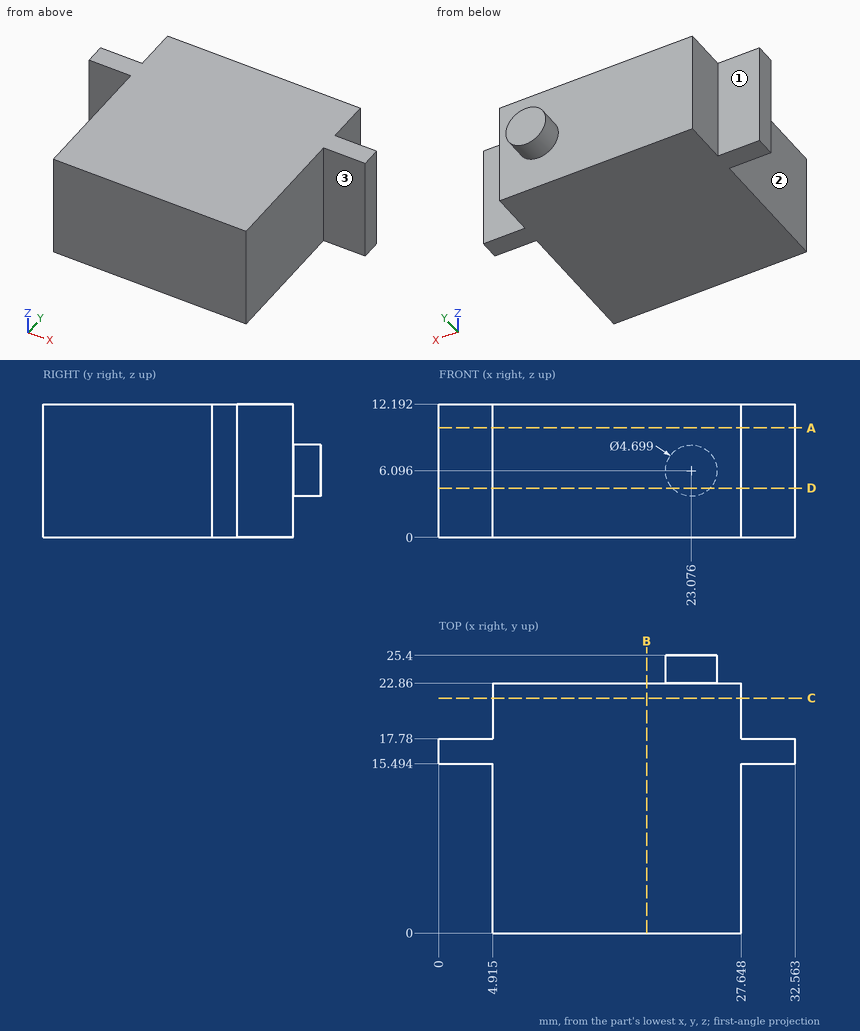
Print and shaded views of the part. All mm, measured from the part's lowest x, y and z. A direction names the side the tool comes from. Coordinates: 2 decimals unless noted, no trailing zeros. Write each loop counter-clockwise with the first axis right and the second up, starting at its lowest first coordinate (ties: lowest second). Pieces come first, ordered by that corner, then holes. Notation, with made-up numbers: M 7,22.25 L 24,22.25 A26 cw 24,56.25 Z; hole C 54.5,23 d5. An arc over 180 degrees is marked long. Return JSON: item names as keys, results as strings.
1. 3-axis set-ups, long thin cutter, end or side, ignore diameter. For the marked faces 1, 2 and 3: which of +Z, -Z, +X, -X, +Y, -Y reach the whole face in a straight line?
Determined:
{"face 1": "+Z, -Z, -X, +Y", "face 2": "+Z, -Z, -X, -Y", "face 3": "+Z, -Z, +X, -Y"}
2. Probe L1, parallel to X at y = 8.75, z = 1.5 (1 decimal); L2, parallel to Y at x = 17, z = 9.25; L3, parallel to Y at x = 29, z = 7.25. List the from-to ranges inside material, lowest first.
Determined:
{"L1": "4.9 to 27.6", "L2": "0 to 22.86", "L3": "15.49 to 17.78"}
3. Saw through at B-B, the plane x = 19. Write the cut outline in (y, z), then the cut area to 3 significant figures.
Determined:
{"outline": "M 0,0 L 22.86,0 L 22.86,12.19 L 0,12.19 Z", "area": "279 mm²"}
4. Saw through at A-A, the plane z = 10. Write the cut outline in (x, y) (1 decimal).
Determined:
{"outline": "M 0,15.5 L 4.9,15.5 L 4.9,0 L 27.6,0 L 27.6,15.5 L 32.6,15.5 L 32.6,17.8 L 27.6,17.8 L 27.6,22.9 L 4.9,22.9 L 4.9,17.8 L 0,17.8 Z"}
5. Flat gauge pins, fed straight in: pin 1 Ø10 at (x, y) = (28.5, 7.5) entering from +Z; pin 2 Ø2.5 at (y, z) = (21, 6.5) entering from +X; pin 3 Ø2.5 at (x, z) = (3.5, 6.5) entering from +Y; pin 4 Ø4 at (x, z) = (2.5, 6) entering from -Y. Where does each tip first touch, or does it go through?
Determined:
{"pin 1": "z = 12.19", "pin 2": "x = 27.65", "pin 3": "y = 17.78", "pin 4": "y = 15.49"}
6. Saw through at D-D, the plane z = 4.5. Write the cut outline in (x, y) (1 decimal), then the cut area to 3 significant figures.
Determined:
{"outline": "M 0,15.5 L 4.9,15.5 L 4.9,0 L 27.6,0 L 27.6,15.5 L 32.6,15.5 L 32.6,17.8 L 27.6,17.8 L 27.6,22.9 L 24.8,22.9 L 24.8,25.4 L 21.4,25.4 L 21.4,22.9 L 4.9,22.9 L 4.9,17.8 L 0,17.8 Z", "area": "551 mm²"}
7. Saw through at C-C, the plane y = 21.5. Write the cut outline in (x, z) (1 decimal), then the cut area to 3 significant figures.
Determined:
{"outline": "M 4.9,0 L 27.6,0 L 27.6,12.2 L 4.9,12.2 Z", "area": "277 mm²"}
